Solid Edge part; units mm, degrees
sketch "Sketch1" plane through (0, 0, 0) normal (0, 0, 1) x (1, 0, 0)
  line L0 (-47.5, -28) -> (47.5, -28)
  line L1 (47.5, -28) -> (47.5, 28)
  line L2 (47.5, 28) -> (-47.5, 28)
  line L3 (-47.5, 28) -> (-47.5, -28)
  line L4 (-56.2504, -36.5) -> (56, -36.5)
  line L5 (56, -36.5) -> (56, 36.5)
  line L6 (56, 36.5) -> (-56.2504, 36.5)
  line L7 (-56.2504, 36.5) -> (-56.2504, -36.5)
  circle A0 centre (-52.0004, 32.25) radius 1.5
  circle A1 centre (0, 32.25) radius 1.5
  circle A2 centre (51.75, 32.25) radius 1.5
  circle A3 centre (51.75, 0) radius 1.5
  circle A4 centre (51.75, -32.25) radius 1.5
  circle A5 centre (-52.0004, -32.25) radius 1.5
  circle A6 centre (-2.4598, -32.5922) radius 1.5
  circle A7 centre (-52.0004, 0) radius 1.5
  dimension "D1" = 47.5
  dimension "D2" = 47.5
extrude "ProtrusiónExtruida_15" add sketch "Sketch1" along normal blind 1.5
Geometry: final body of the model. Coordinates: model frame, mm. Coordinates: 2 decimals unless noted, no trailing zeros. Write each loop counter-clockwise with the first axis right and the second up, starting at its lowest first coordinate (ties: lowest second). Pieces come first, ordered by that corner, then holes. Notation, with made-up numbers: (89.5, 0.5) - (109.5, 0.5) arc R34 ccw to (109.5, 31.5) - close; hole circle Ø11 at (-18.75, -17). An arc over 180 degrees is marked (long way). Return JSON: item names as keys, results as strings.
Item 1: Section query B-B (y = 0). Output: boundary loops of the cut face in (x, z).
Completed:
{"outline": "(-56.25, 0) - (-53.5, 0) - (-53.5, 1.5) - (-56.25, 1.5) - close; (-50.5, 0) - (-47.5, 0) - (-47.5, 1.5) - (-50.5, 1.5) - close; (47.5, 0) - (50.25, 0) - (50.25, 1.5) - (47.5, 1.5) - close; (53.25, 0) - (56, 0) - (56, 1.5) - (53.25, 1.5) - close"}
Item 2: Pull-direction query (Y, two-part tool) for faces 1 (the face through (-50.615, 32.825, 0.74)), 2 (the face through (-2.785, -31.128, 0.74)), 3 (the face through (0, 30, 0)); classes: +Y half, -Y half, draft (parallel to the pull), parting line (faces both ways), or undercut.
Completed:
{"face 1": "undercut", "face 2": "undercut", "face 3": "draft"}
Item 3: Section query D-D (z = 0.65). Count the separate pieces of the cut face and the enclosed holes in it, and give its area (3 significant figures).
Completed:
{"separate pieces": "1", "enclosed holes": "9", "area": "2,820 mm2"}
Item 4: Line query: L1, parallel to Y at x = 51.5, z = 0.15; L2, parallel to Y at x = 43.5, z = 1.45; L3, parallel to X at y = -11, z = 0.4. Output: solid intervals per line, ascending.
Completed:
{"L1": "y = -36.5 to -33.73, -30.77 to -1.48, 1.48 to 30.77, 33.73 to 36.5", "L2": "y = -36.5 to -28, 28 to 36.5", "L3": "x = -56.25 to -47.5, 47.5 to 56"}
Item 5: Section query C-C (x = 51.75). Output: boundary loops of the cut face in (y, z), and give its area (3 significant figures).
Completed:
{"outline": "(-36.5, 0) - (-33.75, 0) - (-33.75, 1.5) - (-36.5, 1.5) - close; (-30.75, 0) - (-1.5, 0) - (-1.5, 1.5) - (-30.75, 1.5) - close; (1.5, 0) - (30.75, 0) - (30.75, 1.5) - (1.5, 1.5) - close; (33.75, 0) - (36.5, 0) - (36.5, 1.5) - (33.75, 1.5) - close", "area": "96.0 mm2"}
Item 6: Section query A-A (y = 11). Output: boundary loops of the cut face in (x, z).
Completed:
{"outline": "(-56.25, 0) - (-47.5, 0) - (-47.5, 1.5) - (-56.25, 1.5) - close; (47.5, 0) - (56, 0) - (56, 1.5) - (47.5, 1.5) - close"}
